```python
from build123d import *

# Parameters (mm, degrees)
BLANKSKE_W         = 150
BLANKSKE_H         = 12
BLANK_DEPTH        = 10
TOOTHCUTSIM_DEPTH  = 151.811140172
TEETHCUTS_COUNT    = 25
TEETHCUTS_PITCH    = 6.2831853
CUT_EXTRUDE1_DEPTH = 6.825


with BuildPart() as part:
    # BlankSke → Blank (new body)
    with BuildSketch(Plane.XY):
        with Locations((75, 6)):
            Rectangle(BLANKSKE_W, BLANKSKE_H)
    extrude(amount=-BLANK_DEPTH)

    # TooCutSkeSim → ToothCutSim (cut, through all)
    with BuildSketch(Plane.XY):
        Polygon((0.861870739, 7.5), (-0.861870739, 7.5), (-2.508981637, 12.0254), (2.508981637, 12.0254), align=None)
    toothcutsim = extrude(amount=-TOOTHCUTSIM_DEPTH, mode=Mode.SUBTRACT)

    # TeethCuts: ToothCutSim ×25
    with Locations(*[(i * TEETHCUTS_PITCH, 0, 0) for i in range(1, TEETHCUTS_COUNT)]):
        add(toothcutsim, mode=Mode.SUBTRACT)

    # Sketch1 → Cut-Extrude1 (cut)
    with BuildSketch(Plane.XY):
        Polygon((150, 7.5), (149.934576461, 7.5), (148.296710406, 12), (147.012998694, 12), (145.375132639, 7.5), (143.651391161, 7.5), (142.013525106, 12), (140.729813394, 12), (139.091947339, 7.5), (137.368205861, 7.5), (135.730339806, 12), (134.446628094, 12), (132.808762039, 7.5), (131.085020561, 7.5), (129.447154506, 12), (128.163442794, 12), (126.525576739, 7.5), (124.801835261, 7.5), (123.163969206, 12), (121.880257494, 12), (120.242391439, 7.5), (118.518649961, 7.5), (116.880783906, 12), (115.597072194, 12), (113.959206139, 7.5), (112.235464661, 7.5), (110.597598606, 12), (109.313886894, 12), (107.676020839, 7.5), (105.952279361, 7.5), (104.314413306, 12), (103.030701594, 12), (101.392835539, 7.5), (99.669094061, 7.5), (98.031228006, 12), (96.747516294, 12), (95.109650239, 7.5), (93.385908761, 7.5), (91.748042706, 12), (90.464330994, 12), (88.826464939, 7.5), (87.102723461, 7.5), (85.464857406, 12), (84.181145694, 12), (82.543279639, 7.5), (80.819538161, 7.5), (79.181672106, 12), (77.897960394, 12), (76.260094339, 7.5), (74.536352861, 7.5), (72.898486806, 12), (71.614775094, 12), (69.976909039, 7.5), (68.253167561, 7.5), (66.615301506, 12), (65.331589794, 12), (63.693723739, 7.5), (61.969982261, 7.5), (60.332116206, 12), (59.048404494, 12), (57.410538439, 7.5), (55.686796961, 7.5), (54.048930906, 12), (52.765219194, 12), (51.127353139, 7.5), (49.403611661, 7.5), (47.765745606, 12), (46.482033894, 12), (44.844167839, 7.5), (43.120426361, 7.5), (41.482560306, 12), (40.198848594, 12), (38.560982539, 7.5), (36.837241061, 7.5), (35.199375006, 12), (33.915663294, 12), (32.277797239, 7.5), (30.554055761, 7.5), (28.916189706, 12), (27.632477994, 12), (25.994611939, 7.5), (24.270870461, 7.5), (22.633004406, 12), (21.349292694, 12), (19.711426639, 7.5), (17.987685161, 7.5), (16.349819106, 12), (15.066107394, 12), (13.428241339, 7.5), (11.704499861, 7.5), (10.066633806, 12), (8.782922094, 12), (7.145056039, 7.5), (5.421314561, 7.5), (3.783448506, 12), (2.499736794, 12), (0.861870739, 7.5), (0, 7.5), (0, 0), (150, 0), align=None)
    extrude(amount=-CUT_EXTRUDE1_DEPTH, mode=Mode.SUBTRACT)


solid = part.part
```
Geometry check sheet. Reference: the model listing, model coordinates, mm. A direction names the side the tool comes from. Coordinates: 2 decimals unless noted, no trailing zeros. One line per item, written item: value. Start each with the question number.
(1) Mould release check, pull along X, two halves, no side actions. Record for faces 3 (the flat face through (149.127, 9.719, -8.39)), 4 (the flat face through (74, 5, -6.825)), 5 (the flat face through (133.64, 9.78, -8.39)), 6 (the flat face through (36.03, 9.72, -8.39)): released by +X, released by -X, zero draft, split by the parting line, or undercut.
(2) Tool access check on faces 1 (the flat face through (74, 5, -10)), 2 (the flat face through (42.313, 9.719, -8.39)). Record the directions out of +Z, -Z, +X, -X, +Y, -Y that give a thin tool (end or side, any length) a straight path to the whole face; none if there is none.
(3) Material ranges on line 1 (Y direction, x = 50, z = -8.7), recorded low to high. Write a range as [from, to].
(4) Depth check by flat-ended pin: P1, Ø1.4, axis at x = 132, z = -8, coming from the +Y side. Enter the tip coordinate at first touch or a pass-through.
Results below:
1. face 3: released by +X
1. face 4: zero draft
1. face 5: undercut
1. face 6: undercut
2. face 1: -Z, +X, -X, +Y, -Y
2. face 2: +Z, -Z, +Y
3. line 1: y = [0, 7.5]
4. P1: stops at y = 7.5
